Verification items for the finished model (mm, model axes). Round coordinates to 2 decimals unless told otherwise and drop trailing zeros. Order: outer loops, then holes, each group sorted by start corner. A loop starts at its lowest first (then second) coordinate and runs counter-clockwise, first axis right, second up. Notation, with made-up numbers: M -11.75,7 L 7.25,7 A28 cw 7.25,38 Z; hole C 36,23.25 d5. An arc over 180 degrees is marked long. Use one line per item in the form item = value. Start each with the question number.
Item 1: Cross-section at C-C on x = -40. Enter the section's corners in (y, z).
Item 2: Thickness scan on probe 1 along X at (y, z) = (33, 31.5); probe 2 along Z at (x, y) = (-24.5, 51.5); probe 3 along Z at (x, y) = (-21, 12.5). Record the ranges inside material, lowest first. Write a range as [from, to].
Item 3: Go/stop test with flat-tipped pins: pin 1 Ø1 at (y, z) = (6, 11) entering from -X; pin 2 Ø10 at (x, z) = (-31.5, -0.5) entering from -Y; pin 3 Ø1 at (y, z) = (27.5, 23.5) entering from -X; pin 4 Ø4 at (x, y) = (-33.5, 45) entering from +Z. Record where each tip stops, or that it passes through.
Item 4: Cross-section at A-A on y = 22.5. Enter the section's corners in (x, z).
Item 5: Cross-section at B-B on z = 26. Enter the section's corners in (x, y).
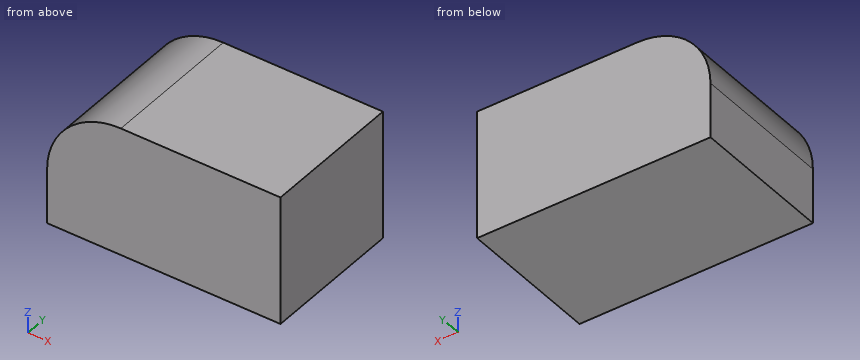
from build123d import *

# Parameters (mm, degrees)
F0_W     = 92.442896
F0_H     = 50.99131
F1_DEPTH = 56.5
F2_R     = 29.211984


with BuildPart() as f1:
    # F0 (on Front) → F1 (new body)
    with BuildSketch(Plane.XZ):
        with Locations((-0.082703, 9.766088)):
            Rectangle(F0_W, F0_H)
    extrude(amount=-F1_DEPTH)

    # F2
    f2_edges = [f1.edges().sort_by_distance(p)[0] for p in [
        (-46.304151, 28.25, 35.261743),
    ]]
    fillet(f2_edges, radius=F2_R)


solid = f1.part
Output values:
q1.outline = M 0,-15.73 L 56.5,-15.73 L 56.5,24.18 L 0,24.18 Z
q2.probe_1 = [-31.43, 46.14]
q2.probe_2 = [-15.73, 34.31]
q2.probe_3 = [-15.73, 35]
q3.pin_1 = -45.96
q3.pin_2 = 0
q3.pin_3 = -40.88
q3.pin_4 = 31.46
q4.outline = M -46.3,-15.73 L 46.14,-15.73 L 46.14,35.26 L -17.09,35.26 A29.21 ccw -46.3,6.05 Z
q5.outline = M -38.43,0 L 46.14,0 L 46.14,56.5 L -38.43,56.5 Z
